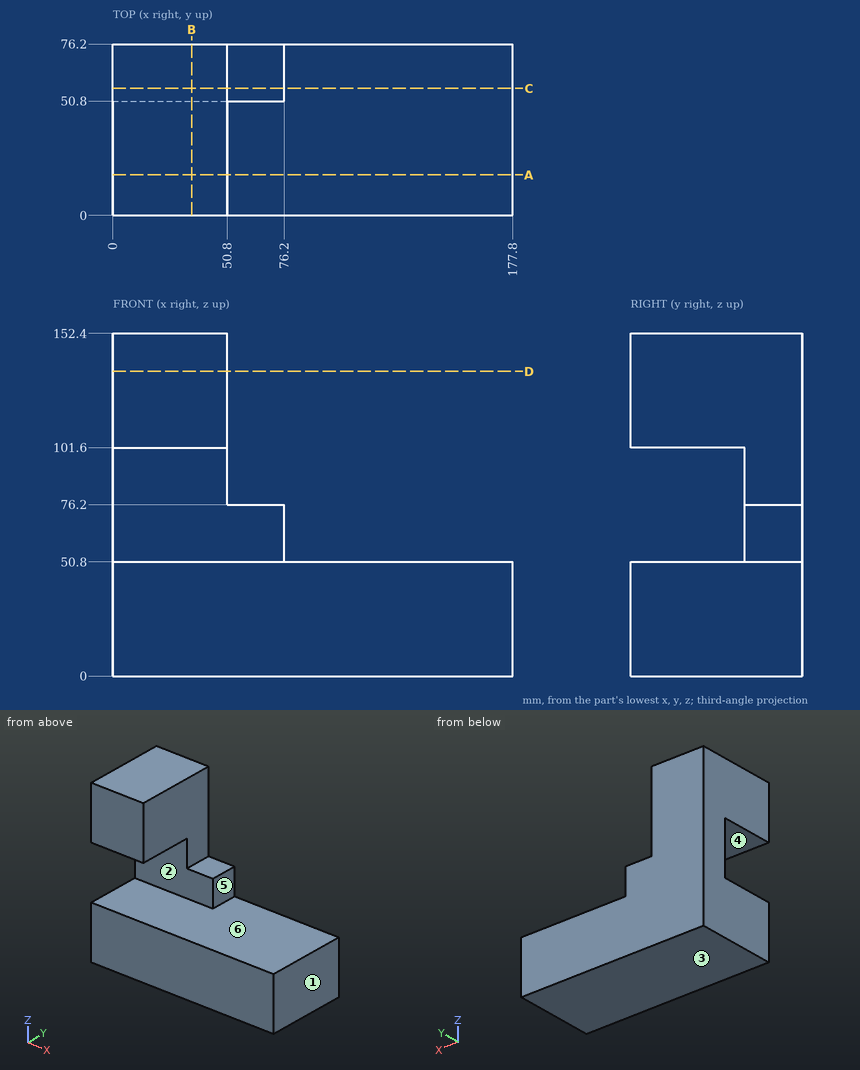
Here's the drawing with two shaded views (mm, measured from the low corner). I have some questions. A direction names the side the tool comes from. Give positions to 0.01 mm unless a question says otherwise; leave off trailing zeros. Order: outer loops, then holes, each group sorted by start corner. A loop starts at its lowest first (then second) coordinate and runs counter-clockwise, first axis right, second up. Notation, with made-up numbers: M 69,19 L 73,19 A23 cw 73,52 Z; hole C 0.5,59 d4. An arc over 180 degrees is marked long. Answer as a JSON object with one key per item and string values. Group by question number.
1) Suppose I cut it at C-C, the plane y = 56.5. Write out the boundary of the cut face in (x, z).
2) Please list where these lines run through material, in increasing order: L1, parallel to X at y = 23.5, z = 112.5; L2, parallel to Y at x = 34.5, z = 83. Write a range as [from, to].
3) On a 3-axis mill with a long thin cutter (end or side, diameter ignored), from which of +Z, -Z, +X, -X, +Y, -Y can I reach the whole of each face in a straight line? I mean the marked faces 4, 5 and 6. Say none if no direction works.
4) Suppose I cut it at A-A, the plane y = 18. Write out the boundary of the cut face in (x, z), plus the area to 3 significant figures.
5) We'd pull the mould along Z, two halves only. Please class the marked faces 1, 2 and 3: pulls with the +Z half, pulls with the -Z half, needs draft (parallel to the pull), parting line crosses it, or undercut.
6) Suppose I cut it at B-B, the plane x = 35. Write out the boundary of the cut face in (y, z), plus the area to 3 significant figures.
7) Suppose I cut it at D-D, the plane z = 135.5. Write out the boundary of the cut face in (x, y), plus the area to 3 significant figures.
8) I'm going to push flat-ended pins straight in: pin 1 Ø8 at (y, z) = (38, 135.5) entering from +X; pin 2 Ø20.5 at (x, y) = (67.5, 68) entering from +Z. Where does each tip first touch, or does it pass through?
Results found:
{
 "1": {"outline": "M 0,0 L 177.8,0 L 177.8,50.8 L 76.2,50.8 L 76.2,76.2 L 50.8,76.2 L 50.8,152.4 L 0,152.4 Z"},
 "2": {"L1": "[0, 50.8]", "L2": "[50.8, 76.2]"},
 "3": {"face 4": "+X, -X, -Y", "face 5": "+Z, +X, +Y, -Y", "face 6": "+X, -Y"},
 "4": {"outline": "M 0,0 L 177.8,0 L 177.8,50.8 L 0,50.8 Z; M 0,101.6 L 50.8,101.6 L 50.8,152.4 L 0,152.4 Z", "area": "11,600 mm²"},
 "5": {"face 1": "needs draft", "face 2": "undercut", "face 3": "pulls with the -Z half"},
 "6": {"outline": "M 0,0 L 76.2,0 L 76.2,152.4 L 0,152.4 L 0,101.6 L 50.8,101.6 L 50.8,50.8 L 0,50.8 Z", "area": "9,030 mm²"},
 "7": {"outline": "M 0,0 L 50.8,0 L 50.8,76.2 L 0,76.2 Z", "area": "3,870 mm²"},
 "8": {"pin 1": "x = 50.8", "pin 2": "z = 76.2"}
}
